Read the model definition and answer for the solid it produces. Units are mm, in the model's axes. Face numbers are marked on the shaded views. Coordinates: 2 decimals unless noted, no trailing zeros. Write each loop counter-clockwise with the first axis right and the second up, starting at its lowest first coordinate (ties: lowest second). Pieces come first, ordered by that corner, then holes. Notation, with made-up numbers: (-5.5, -9.5) - (4.5, -9.5) arc R22 cw to (4.5, 8.5) - close; hole circle Ø2 at (-8, 86). An arc over 180 degrees is marked (long way). Return JSON: item names as keys, results as strings.
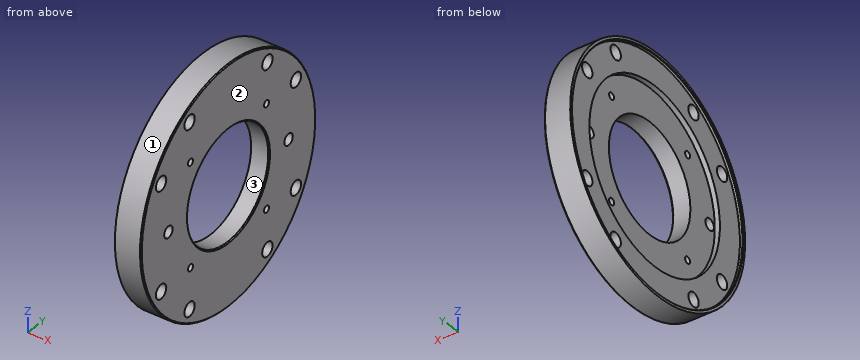
```python
from build123d import *

# Parameters (mm, degrees)
CUT_EXTRUDE_1_DEPTH      = 169.890497068
CUT_EXTRUDE_1_DEPTH_BACK = 169.890497068
SKETCH_2_R               = 7
SKETCH_2_R_2             = 3.4
SKETCH_2_R_3             = 5.7226


with BuildPart() as part:
    # ｽｹｯﾁ1 → 回転1 (revolve)
    with BuildSketch(Plane.XY, mode=Mode.PRIVATE) as revolve_1_sk:
        Polygon((0, 115.5), (0.5, 115), (3, 115), (3, 88), (8, 88), (8, 55), (25, 55), (26, 56), (26, 117), (25, 118), (0, 118), align=None)
    revolve(revolve_1_sk.sketch.rotate(Axis((0, 0, 0), (1, 0, 0)), 90), axis=Axis((0, 0, 0), (1, 0, 0)))

    # ｽｹｯﾁ2 → ｶｯﾄ - 押し出し1 (cut, two sides: drawn at the far end of the back side and taken through both)
    with BuildSketch(Plane(origin=(0, 0, 0), x_dir=(0, 0, -1), z_dir=(1, 0, 0)).offset(-CUT_EXTRUDE_1_DEPTH_BACK)):
        with Locations((90.932667397, 52.5)):
            Circle(SKETCH_2_R)
        with Locations((52.5, 90.932667397)):
            Circle(SKETCH_2_R)
        with Locations((-52.5, 90.932667397)):
            Circle(SKETCH_2_R)
        with Locations((-90.932667397, 52.5)):
            Circle(SKETCH_2_R)
        with Locations((-90.932667397, -52.5)):
            Circle(SKETCH_2_R)
        with Locations((-52.5, -90.932667397)):
            Circle(SKETCH_2_R)
        with Locations((52.5, -90.932667397)):
            Circle(SKETCH_2_R)
        with Locations((90.932667397, -52.5)):
            Circle(SKETCH_2_R)
        with Locations((51.265241636, 51.265241636)):
            Circle(SKETCH_2_R_2)
        with Locations((-51.265241636, 51.265241636)):
            Circle(SKETCH_2_R_2)
        with Locations((-51.265241636, -51.265241636)):
            Circle(SKETCH_2_R_2)
        with Locations((51.265241636, -51.265241636)):
            Circle(SKETCH_2_R_2)
        with Locations((0, 81)):
            Circle(SKETCH_2_R_3)
        with Locations((0, -81)):
            Circle(SKETCH_2_R_3)
    extrude(amount=CUT_EXTRUDE_1_DEPTH + CUT_EXTRUDE_1_DEPTH_BACK, mode=Mode.SUBTRACT)


solid = part.part
```
(1) A cutting plane is placed at A-A (y = 0). Determine the outline of the cut face in (x, z).
Answer:
{"outline": "(0, -118) - (25, -118) - (26, -117) - (26, -56) - (25, -55) - (8, -55) - (8, -88) - (3, -88) - (3, -115) - (0.5, -115) - (0, -115.5) - close; (0, 115.5) - (0.5, 115) - (3, 115) - (3, 88) - (8, 88) - (8, 55) - (25, 55) - (26, 56) - (26, 117) - (25, 118) - (0, 118) - close"}
(2) A cutting plane is placed at B-B (y = 95). State how many separate pieces and enclosed holes the cut face has, and give its area (3 significant figures).
Answer:
{"separate pieces": "3", "enclosed holes": "0", "area": "2,720 mm²"}
(3) Flat-ended cylindrical pins translate along their axes: P1, Ø1, axis at x = 12, z = -24.5, coming from the -Y side; P2, Ø8, axis at x = 13, z = 73, coming from the +Y side; P3, Ø13, axis at y = 81, z = 0, coming from the -X side; P4, Ø11, axis at y = 51.27, z = -51.27, coming from the +X side. Find the tip coordinate at first contact, or state that the pin passes through.
Answer:
{"P1": "y = -115.53", "P2": "y = 95.72", "P3": "x = 8", "P4": "x = 26"}
(4) Determine the mould class of the marked faces 1, 2 and 3 for opening direction Z: +Z half, -Z half, draft (parallel to the pull), parting line (faces both ways), or undercut.
Answer:
{"face 1": "parting line", "face 2": "draft", "face 3": "undercut"}
(5) Straight lines are drawn through the part: line 1 (Y direction, x = 23.5, z = 0.5); line 2 (Y direction, x = 12.5, z = -84.5); line 3 (Y direction, x = 11.75, z = -85.5). For each, find the intervals that lie inside material, in ascending order. Write a range as from..to.
Answer:
{"line 1": "-118..-86.7, -75.3..-55, 55..75.3, 86.7..118", "line 2": "-82.36..-55.26, -49.74..49.74, 55.26..82.36", "line 3": "-81.32..-56.91, -48.09..48.09, 56.91..81.32"}
